Design review of the part built by this model. Coordinates are the model's own, in mm. A direction names the side the tool comes from. Give positions to 0.01 mm unless a question says otherwise; leave off trailing zeros. Write each loop counter-clockwise with the first axis right and the second up, starting at its lowest first coordinate (ties: lowest second). Pieces come first, ordered by that corner, then holes.
```python
from build123d import *

# Parameters (mm, degrees)
SKETCH3_W           = 13.5
SKETCH3_H           = 10.382914324
BOSS_EXTRUDE1_DEPTH = 9.525
BOSS_EXTRUDE2_START = -14.243138
SKETCH4_W           = 13.5
SKETCH4_H           = 7.234030804
BOSS_EXTRUDE2_DEPTH = 14.243138


with BuildPart() as part:
    # Sketch1 → Revolve1 (revolve)
    with BuildSketch(Plane(origin=(0, 0, 0), x_dir=(0, 0, -1), z_dir=(1, 0, 0))):
        with BuildLine():
            Line((0, 42.48431703), (0, -4.71568297))
            Line((0, -4.71568297), (-4.933645932, -4.71568297))
            Line((-4.933645932, -4.71568297), (-5.5, -1.585086748))
            ThreePointArc((-5.5, -1.585086748), (-6.999396572, 0.043766636), (-5.4125, 1.5875))
            Line((-5.4125, 1.5875), (-6.75, 4.851437808))
            Line((-6.75, 4.851437808), (-6.75, 24.552512087))
            Line((-6.75, 24.552512087), (-6.346345985, 24.552512087))
            Line((-6.346345985, 24.552512087), (-6.346345985, 33.2867))
            Line((-6.346345985, 33.2867), (-5.588, 33.2867))
            Line((-5.588, 33.2867), (-5.588, 34.6075))
            Line((-5.588, 34.6075), (-6.346345985, 34.6075))
            Line((-6.346345985, 34.6075), (-6.346345985, 37.7825))
            Line((-6.346345985, 37.7825), (-5.4125, 37.7825))
            ThreePointArc((-5.4125, 37.7825), (-6.981405369, 39.612264718), (-4.933645932, 40.883557079))
            Line((-4.933645932, 40.883557079), (-4.933645932, 41.654223502))
            Line((-4.933645932, 41.654223502), (-5.880026524, 41.654223502))
            Line((-5.880026524, 41.654223502), (-5.880026524, 42.48431703))
            Line((-5.880026524, 42.48431703), (0, 42.48431703))
        make_face()
    revolve(axis=Axis((0, 42.48431703, 0), (0, -1, 0)))



with BuildPart() as body_2:
    # Sketch3 → Boss-Extrude1 (new body)
    with BuildSketch(Plane(origin=(0, 17.673005927, -17.673005927), x_dir=(1, 0, 0), z_dir=(0, -0.707106781, 0.707106781))):
        with Locations((0, 9.889573108)):
            Rectangle(SKETCH3_W, SKETCH3_H)
    extrude(amount=-BOSS_EXTRUDE1_DEPTH)


with BuildPart() as part_1:
    add(part.part)

    add(body_2.part)  # Boss-Extrude2 merges body 2
    # Sketch4 → Boss-Extrude2 (add)
    with BuildSketch(Plane.XY.offset(BOSS_EXTRUDE2_START)):
        with Locations((0, 24.719889296)):
            Rectangle(SKETCH4_W, SKETCH4_H)
    extrude(amount=BOSS_EXTRUDE2_DEPTH)


solid = part_1.part
```
(1) To check wall thickness, follow L1, parallel to Y at x = 5, z = -4.5; L2, parallel to X at y = 25.5, z = -14; L3, parallel to Y at x = 5.25, z = -7. State the ranges of each line that lie inside material, in increasing order.
Resolved:
L1: y = -0.89 to 0.89, 4.79 to 28.34, 38.48 to 40.26
L2: x = -6.75 to 6.75
L3: y = 21.1 to 28.34
(2) Consider section A-A, the plane z = -12. Give the boundary of the cut face in (x, y).
Resolved:
outline: (-6.75, 21.1) - (6.75, 21.1) - (6.75, 33.33) - (-6.75, 33.33) - close
(3) Mouldability with a two-part tool opening along Z and no side actions: class faces 5 (the face through (4.912, -4.172, -1.091)), 6 (the face through (-0.09, 31.66, -10.33)), 7 (the face through (6, 33.287, 0)), 8 (the face through (6.75, 26, -11)) as pulls with the +Z half, pulls with the -Z half, needs draft (parallel to the pull), parting line crosses it, or undercut.
Resolved:
face 5: parting line crosses it
face 6: undercut
face 7: undercut
face 8: needs draft
(4) Clearance check with flat-ended pins moving along their axes: P1, Ø5, axis at x = -1, y = 0, coming from the -Z side; P2, Ø10, axis at y = 23.5, z = -2, coming from the -X side; P3, Ø10, axis at y = 34.5, z = -3, coming from the -X side. State where each tip first meets the part, or that it passes through.
Resolved:
P1: stops at z = -7
P2: stops at x = -6.75
P3: stops at x = -6.91
(5) Consider section B-B, the plane y = 18. Give the boundary of the cut face in (x, z).
Resolved:
outline: circle Ø13.5 at (0, 0)
(6) Tool access review of faces 1 (the face through (-6.29, 36.22, -0.83)), 2 (the face through (0, 42.484, 0)), 3 (the face through (-4.96, 42.08, 3.16)), 4 (the face through (0, 24.553, 6.6)): name each direction out of +Z, -Z, +X, -X, +Y, -Y from which nothing blocks a thin tool from reaching the whole face with its end or side.
Resolved:
face 1: none
face 2: +Z, -Z, +X, -X, +Y
face 3: +Y
face 4: +Z
